CAD build for the part. Positions are in the model's coordinates, mm. A direction names the side the tool comes from. Round coordinates to 2 decimals unless told otherwise and drop trailing zeros. Order: outer loops, then holes, each group sorted by start corner. A loop starts at its lowest first (then second) coordinate and runs counter-clockwise, first axis right, second up. Notation, with made-up numbers: M 58.25,1 L 82.25,1 A17 cw 82.25,17 Z; hole C 3.5,55.25 d1. An arc over 180 degrees is marked long. Answer as a JSON object with one key per item and string values. Group by question number.
```python
from build123d import *

# Parameters (mm, degrees)
BOSS_EXTRUDE1_OUTLINE_R = 9
BOSS_EXTRUDE1_DEPTH     = 1
SKETCH2_R               = 6.1121977
BOSS_EXTRUDE2_DEPTH     = 3.25
SKETCH3_R               = 2.5
CUT_EXTRUDE1_DEPTH      = 16.305227865
SKETCH4_R               = 5.6
SKETCH4_R_2             = 5.5
SKETCH4_R_3             = 4.5
SKETCH4_R_4             = 3.5
CUT_EXTRUDE2_DEPTH      = 0.5


# Read off the part's stored shape, not the designer's step: Boss-Extrude1
with BuildPart() as part:
    # Boss-Extrude1 outline → Boss-Extrude1 (new body)
    with BuildSketch(Plane(origin=(0, 0, 0), x_dir=(1, 0, 0), z_dir=(0, 1, 0))):
        Circle(BOSS_EXTRUDE1_OUTLINE_R)
    boss_extrude1 = extrude(amount=BOSS_EXTRUDE1_DEPTH)

    # Sketch2 → Boss-Extrude2 (add)
    with BuildSketch(Plane(origin=(0, 1, 0), x_dir=(1, 0, 0), z_dir=(0, 1, 0))):
        with Locations(Location((0, 0, 0), (0, 0, 90))):
            Circle(SKETCH2_R)
    boss_extrude2 = extrude(amount=BOSS_EXTRUDE2_DEPTH)

    # Mirror1: Boss-Extrude2 across plane
    add(boss_extrude2.mirror(Plane.ZX.offset(4.25)))

    # Mirror2: Boss-Extrude1 across plane
    add(boss_extrude1.mirror(Plane.ZX.offset(4.25)))

    # Sketch3 → Cut-Extrude1 (cut, through all)
    with BuildSketch(Plane(origin=(0, 8.5, 0), x_dir=(1, 0, 0), z_dir=(0, 1, 0))):
        with Locations(Location((0, 0, 0), (0, 0, 270))):
            Circle(SKETCH3_R)
    extrude(amount=-CUT_EXTRUDE1_DEPTH, mode=Mode.SUBTRACT)

    # Sketch4 → Cut-Extrude2 (cut)
    # profile 1 of 2: a face of its own
    with BuildSketch(Plane(origin=(0, 8.5, 0), x_dir=(1, 0, 0), z_dir=(0, 1, 0))):
        with Locations(Location((0, 0, 0), (0, 0, 270))):
            Circle(SKETCH4_R)
        with Locations(Location((0, 0, 0), (0, 0, 270))):
            Circle(SKETCH4_R_2, mode=Mode.SUBTRACT)
    # profile 2 of 2: a face of its own
    with BuildSketch(Plane(origin=(0, 8.5, 0), x_dir=(1, 0, 0), z_dir=(0, 1, 0))):
        with Locations(Location((0, 0, 0), (0, 0, 270))):
            Circle(SKETCH4_R_3)
        with Locations(Location((0, 0, 0), (0, 0, 270))):
            Circle(SKETCH4_R_4, mode=Mode.SUBTRACT)
    cut_extrude2 = extrude(amount=-CUT_EXTRUDE2_DEPTH, mode=Mode.SUBTRACT)

    # Mirror3: Cut-Extrude2 across plane
    add(cut_extrude2.mirror(Plane.ZX.offset(4.25)), mode=Mode.SUBTRACT)


solid = part.part
```
Item 1: Two-plate mould, pull along Z, no slides. Class faces 4 (the face through (-2.44, 4.31, -0.54)), 5 (the face through (2, 7.5, 6)), 6 (the face through (-1.172, 0.493, -8.923)): +Z half, -Z half, draft (parallel to the pull), parting line (faces both ways), or undercut.
Item 2: Cut at C-C, the plane y = 6.25. Give the cut face in (x, z).
Item 3: Cut at B-B, the plane x = -7. Give the cut face in (y, z).
Item 4: Cut at A-A, the plane z = 6.5. Give the cut face in (x, y).
Item 5: Flat gauge pins, fed straight in: pin 1 Ø1.5 at (x, y) = (4.5, 7.5) entering from +Z; pin 2 Ø2 at (y, z) = (5.5, -3.5) entering from +X; pin 3 Ø1 at (x, y) = (2.5, 2.5) entering from +Z. Where does each tip first touch, or does it go through?
Item 6: Drill centre lines: line 1 (Y direction, x = -0.75, z = 6.25); line 2 (X direction, y = 4.75, z = 0); line 3 (Z direction, x = -2.25, y = 2). Where is each one in solid material? Low to high. Write a range as [from, to].
Item 7: 3-axis set-ups, long thin cutter, end or side, ignore diameter. For faces 1 (the face through (1.352, 8.254, 4.292)), 2 (the face through (2, 1, 6)), 3 (the face through (1.352, 0.246, 4.292)): which of +Z, -Z, +X, -X, +Y, -Y reach the whole face in a straight line?
Response values:
{
 "1": {"face 4": "undercut", "face 5": "draft", "face 6": "parting line"},
 "2": {"outline": "C 0,0 d12.22; hole C 0,0 d5"},
 "3": {"outline": "M 0,-5.66 L 1,-5.66 L 1,5.66 L 0,5.66 Z; M 7.5,-5.66 L 8.5,-5.66 L 8.5,5.66 L 7.5,5.66 Z"},
 "4": {"outline": "M -6.22,0 L 6.22,0 L 6.22,1 L -6.22,1 Z; M -6.22,7.5 L 6.22,7.5 L 6.22,8.5 L -6.22,8.5 Z"},
 "5": {"pin 1": "z = 8.18", "pin 2": "x = 5.58", "pin 3": "z = 5.78"},
 "6": {"line 1": "[0, 1], [7.5, 8.5]", "line 2": "[-6.11, -2.5], [2.5, 6.11]", "line 3": "[-5.68, -1.09], [1.09, 5.68]"},
 "7": {"face 1": "+Y", "face 2": "none", "face 3": "-Y"}
}
